Part model, mm, in its own coordinate system. A direction names the side the tool comes from. Give positions to 0.01 mm unless a question says otherwise; leave off trailing zeros. Write each loop counter-clockwise with the first axis right and the second up, starting at its lowest first coordinate (ties: lowest second). Pieces come first, ordered by that corner, then holes.
```python
from build123d import *

# Parameters (mm, degrees)
SKETCH_1_W          = 14
SKETCH_1_H          = 8
EXTRUDE_1_DEPTH     = 15
EXTRUDE_2_DEPTH     = 10
SKETCH_4_R          = 2.25
CUT_EXTRUDE_1_DEPTH = 5.5
EXTRUDE_3_DEPTH     = 4


with BuildPart() as part:
    # 草图1 → 凸台-拉伸1 (new body)
    with BuildSketch(Plane(origin=(0, 0, 0), x_dir=(1, 0, 0), z_dir=(0, 1, 0))):
        Polygon((0, 0), (0, 10), (18, 10), (18, -2), (0, -20), align=None)
        with Locations((9, 4)):
            Rectangle(SKETCH_1_W, SKETCH_1_H, mode=Mode.SUBTRACT)
    extrude(amount=EXTRUDE_1_DEPTH)

    # 草图2 → 凸台-拉伸2 (add)
    with BuildSketch(Plane(origin=(0, 15, 0), x_dir=(1, 0, 0), z_dir=(0, 1, 0))):
        Polygon((11.272196348, -3.070949403), (14.100623473, -5.899376527), (7.734731659, -12.265268341), (4.906304534, -9.436841216), align=None)
    extrude(amount=EXTRUDE_2_DEPTH)

    # 草图4 → 切除-拉伸1 (cut)
    with BuildSketch(Plane(origin=(7.171572875, 0, 7.171572875), x_dir=(-0.707106781, 0, 0.707106781), z_dir=(-0.707106781, 0, -0.707106781))):
        with Locations((-1, 21)):
            Circle(SKETCH_4_R)
    extrude(amount=-CUT_EXTRUDE_1_DEPTH, mode=Mode.SUBTRACT)

    # 草图5 → 凸台-拉伸3 (add)
    with BuildSketch(Plane(origin=(10, 0, 10), x_dir=(0.707106781, 0, -0.707106781), z_dir=(0.707106781, 0, 0.707106781))):
        Polygon((5.799157329, 25), (5.799157329, 15), (8.556432914, 15), align=None)
        Polygon((-3.20357321, 25), (-3.20357321, 15), (-6.25343363, 15), align=None)
    extrude(amount=-EXTRUDE_3_DEPTH)


solid = part.part
```
1) Pin check, flat tips, straight feed: pin 1 Ø2 at (y, z) = (6.5, 4.5) entering from +X; pin 2 Ø10 at (x, z) = (3.5, -3) entering from +Y; pin 3 Ø5 at (x, y) = (9, 8.5) entering from +Z. Stop position of each tip, or through.
Answers follow:
pin 1: stops at x = 16.5
pin 2: stops at y = 15
pin 3: stops at z = 13.5
2) Wall check: L1, parallel to X at y = 13.5, z = -0.75; L2, parallel to Z at x = 7, y = 4.75; L3, parallel to Y at x = 2, z = 9.75. Give the ranges that are in metal, low to high.
Answers follow:
L1: x = 0 to 2, 16 to 18
L2: z = -10 to -8, 0 to 13
L3: y = 0 to 15
3) Two-plate mould, pull along Z, no slides. Class faces 3 (the face through (9, 7, -10)), 4 (the face through (5.247, 19.93, 11.964)), 5 (the face through (2, 7, -4)): +Z half, -Z half, draft (parallel to the pull), parting line (faces both ways), or undercut.
Answers follow:
face 3: -Z half
face 4: +Z half
face 5: undercut
4) Saw through at C-C, the plane y = 7.25. Write the cut outline in (x, z), then the cut area to 3 significant figures.
Answers follow:
outline: (0, -10) - (18, -10) - (18, 2) - (0, 20) - close; hole (2, -8) - (16, -8) - (16, 0) - (2, 0) - close
area: 266 mm2
5) Saw through at D-D, the plane x = 1.5. Write the cut outline in (y, z).
Answers follow:
outline: (0, -10) - (15, -10) - (15, 18.5) - (0, 18.5) - close
6) Saw through at A-A, the plane z = -3. Write the cut outline in (x, y), then the cut area to 3 significant figures.
Answers follow:
outline: (0, 0) - (2, 0) - (2, 15) - (0, 15) - close; (16, 0) - (18, 0) - (18, 15) - (16, 15) - close
area: 60.0 mm2
7) 3-axis set-ups, long thin cutter, end or side, ignore diameter. For faces 1 (the face through (9, 7, 0)), 2 (the face through (9, 10, 11)): which of +Z, -Z, +X, -X, +Y, -Y reach the whole face in a straight line?
Answers follow:
face 1: +Y, -Y
face 2: +Z, +X, +Y, -Y
8) Saw through at B-B, the plane y = 20.25. Write the cut outline in (x, z).
Answers follow:
outline: (3.88, 10.46) - (6.38, 7.96) - (9.21, 10.79) - (6.71, 13.29) - close; (9.38, 4.96) - (12.2, 2.14) - (15.03, 4.97) - (12.21, 7.79) - close
